Verification items for the finished model (mm, model axes). Face numbers are marked on the shaded views. Round coordinates to 2 decimals unless told otherwise and drop trailing zeros. Order: outer loops, then holes, each group sorted by start corner. A loop starts at its lowest first (then second) coordinate and runs counter-clockwise, first axis right, second up. Notation, with made-up numbers: (76.25, 36) -> (131.25, 36) arc R18 ccw to (131.25, 63) -> close; hole circle Ø7 at (-37.75, -31.75). An arc over 180 degrees is marked (long way). Return JSON: item names as keys, results as strings. Group by question number.
Item 1: Depth check by flat-ended pin: pin 1 Ø5 at (x, z) = (22, 99) entering from +Y; pin 2 Ø10 at (y, z) = (2.5, 81.5) entering from +X; pin 3 Ø12 at (x, z) = (-9.5, 30) entering from +Y. Enter the tip coordinate at first touch or a pass-through.
Item 2: Sectioned sample at D-D on y = 16. Record the cut outline in (x, z), plus the area to 3 significant figures.
Item 3: Sectioned sample at A-A on y = 0. Record the cut outline in (x, z).
Item 4: Sectioned sample at C-C on x = -13.5. Record the cut outline in (y, z).
Item 5: Draft check along Z on the marked faces 1, 2 and 3. Enter one of: pulls with the +Z half, pulls with the -Z half, needs draft (parallel to the pull), parting line crosses it, or undercut.
Item 6: Scan lines: probe 1 along Z at (x, y) = (-19, 25); probe 2 along Y at (x, z) = (0, 127.5); probe 3 along Y at (x, z) = (-13, 83). Record each from-to range of solid material in increasing order. Write a range as from..to.
Item 7: Sectioned sample at B-B on x = 7. Record the cut outline in (y, z) (3 decimals), plus the area to 3 significant figures.
```python
from build123d import *

# Parameters (mm, degrees)
SKETCH1_R           = 25
SKETCH1_R_2         = 20
BOSS_EXTRUDE2_DEPTH = 200
SKETCH4_R           = 35
SKETCH4_R_2         = 10
BOSS_EXTRUDE3_DEPTH = 10
BOSS_EXTRUDE4_START = 10
SKETCH5_R           = 35
SKETCH5_R_2         = 10
BOSS_EXTRUDE4_DEPTH = 10


with BuildPart() as part:
    # Sketch1 → Boss-Extrude2 (new body)
    with BuildSketch(Plane.XY):
        Circle(SKETCH1_R)
        Circle(SKETCH1_R_2, mode=Mode.SUBTRACT)
    extrude(amount=BOSS_EXTRUDE2_DEPTH)

    # Sketch4 → Boss-Extrude3 (add)
    with BuildSketch(Plane.XY.offset(200)):
        Circle(SKETCH4_R)
        Circle(SKETCH4_R_2, mode=Mode.SUBTRACT)
    extrude(amount=BOSS_EXTRUDE3_DEPTH)

    # Sketch5 → Boss-Extrude4 (add)
    with BuildSketch(Plane(origin=(0, 0, 0), x_dir=(-1, 0, 0), z_dir=(0, 0, -1)).offset(BOSS_EXTRUDE4_START)):
        with Locations(Location((0, 0, 0), (0, 0, 180))):
            Circle(SKETCH5_R)
        with Locations(Location((0, 0, 0), (0, 0, 180))):
            Circle(SKETCH5_R_2, mode=Mode.SUBTRACT)
    extrude(amount=-BOSS_EXTRUDE4_DEPTH)


solid = part.part
```
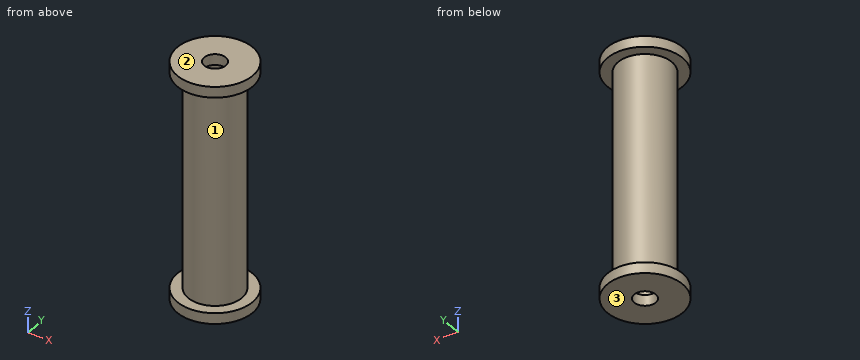
Recorded:
{
 "1": {"pin 1": "y = 15.64", "pin 2": "x = 25", "pin 3": "y = 24.75"},
 "2": {"outline": "(-31.13, -10) -> (31.13, -10) -> (31.13, 0) -> (19.21, 0) -> (19.21, 200) -> (31.13, 200) -> (31.13, 210) -> (-31.13, 210) -> (-31.13, 200) -> (-19.21, 200) -> (-19.21, 0) -> (-31.13, 0) -> close; hole (-12, 0) -> (12, 0) -> (12, 200) -> (-12, 200) -> close", "area": "4,130 mm²"},
 "3": {"outline": "(-35, -10) -> (-10, -10) -> (-10, 0) -> (-20, 0) -> (-20, 200) -> (-10, 200) -> (-10, 210) -> (-35, 210) -> (-35, 200) -> (-25, 200) -> (-25, 0) -> (-35, 0) -> close; (10, -10) -> (35, -10) -> (35, 0) -> (25, 0) -> (25, 200) -> (35, 200) -> (35, 210) -> (10, 210) -> (10, 200) -> (20, 200) -> (20, 0) -> (10, 0) -> close"},
 "4": {"outline": "(-32.29, -10) -> (32.29, -10) -> (32.29, 0) -> (21.04, 0) -> (21.04, 200) -> (32.29, 200) -> (32.29, 210) -> (-32.29, 210) -> (-32.29, 200) -> (-21.04, 200) -> (-21.04, 0) -> (-32.29, 0) -> close; hole (-14.76, 0) -> (14.76, 0) -> (14.76, 200) -> (-14.76, 200) -> close"},
 "5": {"face 1": "undercut", "face 2": "pulls with the +Z half", "face 3": "pulls with the -Z half"},
 "6": {"probe 1": "-10..0, 200..210", "probe 2": "-25..-20, 20..25", "probe 3": "-21.35..-15.2, 15.2..21.35"},
 "7": {"outline": "(-34.293, -10) -> (-7.141, -10) -> (-7.141, 0) -> (-18.735, 0) -> (-18.735, 200) -> (-7.141, 200) -> (-7.141, 210) -> (-34.293, 210) -> (-34.293, 200) -> (-24, 200) -> (-24, 0) -> (-34.293, 0) -> close; (7.141, -10) -> (34.293, -10) -> (34.293, 0) -> (24, 0) -> (24, 200) -> (34.293, 200) -> (34.293, 210) -> (7.141, 210) -> (7.141, 200) -> (18.735, 200) -> (18.735, 0) -> (7.141, 0) -> close", "area": "3,190 mm²"}
}
